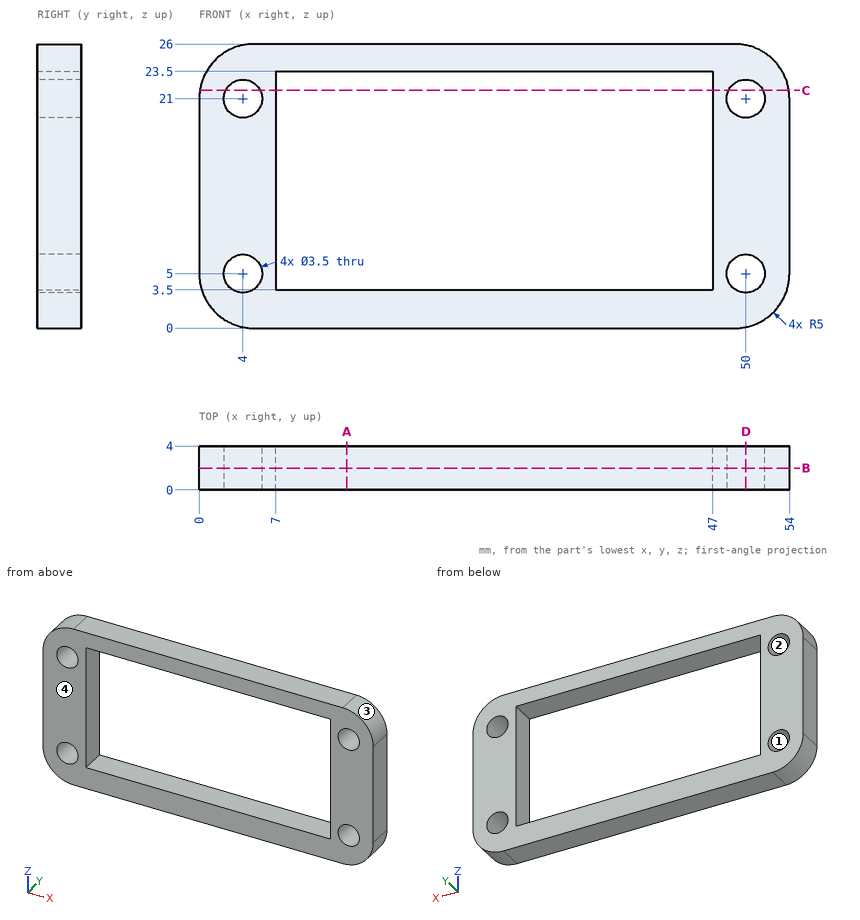
Design review of the part shown in the three views and the two pictorial views. Dimensions are in mm from the part's minimum x, y and z. Coordinates: 2 decimals unless noted, no trailing zeros. Order: outer loops, then holes, each group sorted by start corner. A loop starts at its lowest first (then second) coordinate and runs counter-clockwise, first axis right, second up.
1) Wall thickness on line 1 along X through (y, z) = (1.25, 21); line 2 along Z through (x, y) = (12, 0.9); line 3 along X through (y, z) = (1.05, 11): over which ranges is each line inside the solid? List them lowest first.
2) Take a section at A-A, the plane x = 13.5. Give the boundary of the cut face in (y, z), and give its area (3 significant figures).
3) Mouldability with a two-part tool opening along Z and no side actions: class the marked faces 1, 2, 3 and 4 as +Z half, -Z half, draft (parallel to the pull), parting line (faces both ways), or undercut.
4) Take a section at D-D, the plane x = 50. Give the boundary of the cut face in (y, z).
5) Take a section at C-C, the plane z = 21.75. Give the boundary of the cut face in (x, y), and give its area (3 significant figures).
6) Take a section at B-B, the plane y = 2. Give the boundary of the cut face in (x, z).
7) Clearance check with a flat-ended pin moving along its axis: pin 1 (5 mm diameter, centred on x = 10, z = 9, fed in from +Y). State where the tip first meets the part, or that it passes through.
Returned:
1. line 1: x = 0 to 2.25, 5.75 to 7, 47 to 48.25, 51.75 to 54
1. line 2: z = 0 to 3.5, 23.5 to 26
1. line 3: x = 0 to 7, 47 to 54
2. outline: (0, 0) - (4, 0) - (4, 3.5) - (0, 3.5) - close; (0, 23.5) - (4, 23.5) - (4, 26) - (0, 26) - close
2. area: 24.0 mm2
3. face 1: undercut
3. face 2: undercut
3. face 3: +Z half
3. face 4: draft
4. outline: (0, 0.1) - (4, 0.1) - (4, 3.25) - (0, 3.25) - close; (0, 6.75) - (4, 6.75) - (4, 19.25) - (0, 19.25) - close; (0, 22.75) - (4, 22.75) - (4, 25.9) - (0, 25.9) - close
5. outline: (0.06, 0) - (2.42, 0) - (2.42, 4) - (0.06, 4) - close; (5.58, 0) - (7, 0) - (7, 4) - (5.58, 4) - close; (47, 0) - (48.42, 0) - (48.42, 4) - (47, 4) - close; (51.58, 0) - (53.94, 0) - (53.94, 4) - (51.58, 4) - close
5. area: 30.2 mm2
6. outline: (0, 5) arc R5 ccw to (5, 0) - (49, 0) arc R5 ccw to (54, 5) - (54, 21) arc R5 ccw to (49, 26) - (5, 26) arc R5 ccw to (0, 21) - close; hole circle Ø3.5 at (4, 5); hole circle Ø3.5 at (4, 21); hole (7, 3.5) - (47, 3.5) - (47, 23.5) - (7, 23.5) - close; hole circle Ø3.5 at (50, 5); hole circle Ø3.5 at (50, 21)
7. pin 1: passes through
